Build history of the part. All positions in model axes, mm. Face numbers are marked on the shaded views. Coordinates: 2 decimals unless noted, no trailing zeros. Order: outer loops, then holes, each group sorted by start corner. A loop starts at its lowest first (then second) coordinate and runs counter-clockwise, first axis right, second up. Notation, with made-up numbers: (14.25, 58) - (27.25, 58) arc R33 ccw to (27.25, 97) - close; hole circle Ø5 at (-33.75, 21). An arc over 180 degrees is marked (long way). Write each question's results on one line, items separated by ' | '.
Autodesk Inventor part; units mm, degrees
ref_plane "YZ Plane" through (0, 0, 0) normal (1, 0, 0) x (0, 1, 0)
ref_plane "XZ Plane" through (0, 0, 0) normal (0, 1, 0) x (-1, 0, 0)
ref_plane "XY Plane" through (0, 0, 0) normal (0, 0, 1) x (1, 0, 0)
sketch "Sketch1" plane through (0, 0, 0) normal (0, 0, 1) x (1, 0, 0)
  line L0 (10.7104, 9.7791) -> (42.7104, 9.7791)
  line L1 (42.7104, 9.7791) -> (42.7104, 24.7791)
  line L2 (10.7104, 9.7791) -> (10.7104, 24.7791)
  line L3 (8.7104, 24.7791) -> (8.7104, 7.7791)
  line L4 (8.7104, 7.7791) -> (44.7104, 7.7791)
  line L5 (44.7104, 7.7791) -> (44.7104, 24.7791)
  line L6 (8.7104, 24.7791) -> (10.7104, 24.7791)
  line L7 (42.7104, 24.7791) -> (44.7104, 24.7791)
  point P0 (0, 0)
  dimension "d0" = 32
  dimension "d1" = 15
  dimension "d2" = 15
  dimension "d3" = 2
extrude "Extrusion1" add sketch "Sketch1" along normal blind 100 and the other way blind 5
sketch "Sketch3" plane through (10.7104, 9.7791, 100) normal (0, 1, 0) x (1, 0, 0)
  line L0 (-2, 105) -> (-2, 0)
  line L1 (-2, 91.8971) -> (-2, 105)
  line L2 (32, 105) -> (34, 105)
  line L3 (34, 105) -> (-2, 91.8971)
  line L4 (-2, 105) -> (-2, 91.8971)
  line L5 (-2, 105) -> (34, 105)
  line L6 (0, 105) -> (0, 0)
  line L7 (0, 92.625) -> (0, 105)
  line L8 (34, 105) -> (-2, 99.9405)
  line L9 (34, 105) -> (70.3538, 105) construction
  line L10 (-2, 99.9405) -> (-2, 105)
  point P0 (-10.7104, 100)
  point P1 (-2, 99.9405)
  point P2 (0, 100.2216)
  dimension "d15" = 20
  dimension "d16" = 172
extrude "Extrusion4" cut sketch "Sketch3" along normal through all both and the other way through all contours L5 L6 L8 L0 | L5 L2 L8 L6
extrude "Extrusion5" cut sketch "Sketch3" along normal through all both and the other way through all contours L8 L6 L3 L0
equation "\"BendRadius\" = Thickness"
equation "\"BendReliefWidth\" = Thickness"
equation "\"BendReliefDepth\" = 0.5 * Thickness"
equation "\"CornerReliefSize\" = 4 * Thickness"
equation "\"MinimumRemnant\" = 2 * Thickness"
equation "\"TransitionRadius\" = BendRadius"
equation "\"JacobiRadiusSize\" = BendRadius"
equation "\"GapSize\" = Thickness"
properties part number "outslide"
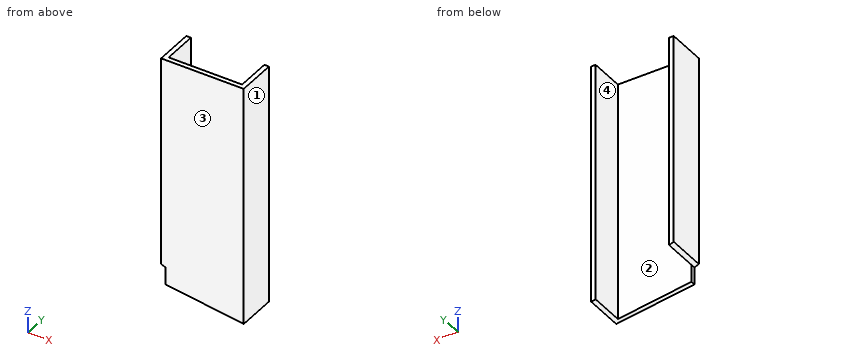
1. Probe line 1 (X direction, y = 15.75, z = 33); line 2 (Y direction, x = 12, z = 8); line 3 (Z direction, x = 43, y = 10). List the from-to ranges inside material, lowest first.
Solved:
line 1: x = 8.71 to 10.71, 42.71 to 44.71 | line 2: y = 7.78 to 9.78 | line 3: z = -4.76 to 100
2. Band-saw the part on C-C on x = 40. Give the cut face in (y, z).
Solved:
outline: (7.78, -4.34) - (9.78, -4.34) - (9.78, 100) - (7.78, 100) - close
3. Drop flat-ended pins along their axis: pin 1 Ø10 at (x, y) = (39, 18) entering from -Z; pin 2 Ø1 at (x, z) = (29, 20.5) entering from +Y; pin 3 Ø1 at (y, z) = (9, 5) entering from -X. Give the stop position or say it passes through.
Solved:
pin 1: stops at z = -4.9 | pin 2: stops at y = 9.78 | pin 3: stops at x = 10.71
4. Band-saw the part on B-B on z = 90. Give the cut face in (x, y).
Solved:
outline: (8.71, 7.78) - (44.71, 7.78) - (44.71, 24.78) - (42.71, 24.78) - (42.71, 9.78) - (10.71, 9.78) - (10.71, 24.78) - (8.71, 24.78) - close
5. Two-plate mould, pull along X, no slides. Class the marked faces 1, 2, 3 and 4: +X half, -X half, draft (parallel to the pull), parting line (faces both ways), or undercut.
Solved:
face 1: +X half | face 2: undercut | face 3: draft | face 4: undercut
6. Band-saw the part on A-A on y = 18. Give the cut face in (x, z) (3 decimals), then the cut area to 3 significant figures.
Solved:
outline: (8.71, 8.103) - (10.71, 7.375) - (10.71, 100) - (8.71, 100) - close; (42.71, -4.719) - (44.71, -5) - (44.71, 100) - (42.71, 100) - close | area: 394 mm2
7. Band-saw the part on D-D on x = 16. Give the cut face in (y, z) (3 decimals).
Solved:
outline: (7.779, -0.965) - (9.779, -0.965) - (9.779, 100) - (7.779, 100) - close
